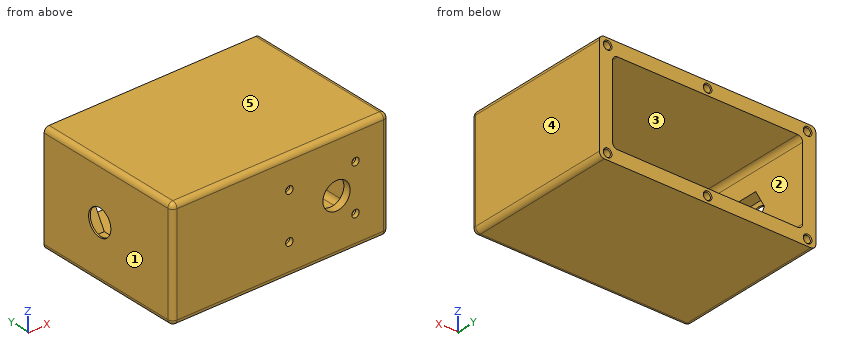
from build123d import *

# Parameters (mm, degrees)
SKETCH1_W           = 131
SKETCH1_H           = 66
BOSS_EXTRUDE1_DEPTH = 92
SKETCH10_W          = 115
SKETCH10_H          = 50
CUT_EXTRUDE7_DEPTH  = 87.5
SKETCH2_R           = 2.25
CUT_EXTRUDE1_DEPTH  = 171.801785705
SKETCH3_R           = 5
CUT_EXTRUDE2_DEPTH  = 171.801785705
SKETCH6_R           = 2.1
CUT_EXTRUDE5_DEPTH  = 7.4
CUT_EXTRUDE9_REACH  = 183.246
SKETCH17_R          = 8
SKETCH19_R          = 1.5
CUT_EXTRUDE12_DEPTH = 20
CUT_EXTRUDE13_DEPTH = 7
SKETCH7_R           = 8.25
SKETCH7_R_2         = 5
CUT_EXTRUDE14_DEPTH = 4.5
SKETCH24_R          = 3.25
CUT_EXTRUDE15_DEPTH = 2
FILLET1_R           = 3
CHAMFER1_SIZE       = 0.5


with BuildPart() as part:
    # Sketch1 → Boss-Extrude1 (new body)
    with BuildSketch(Plane(origin=(0, 0, 0), x_dir=(1, 0, 0), z_dir=(0, 1, 0))):
        with Locations((65.5, -33)):
            Rectangle(SKETCH1_W, SKETCH1_H)
    extrude(amount=BOSS_EXTRUDE1_DEPTH)

    # Sketch10 → Cut-Extrude7 (cut)
    with BuildSketch(Plane(origin=(0, 92, 0), x_dir=(1, 0, 0), z_dir=(0, 1, 0))):
        with Locations((65.5, -33)):
            Rectangle(SKETCH10_W, SKETCH10_H)
    extrude(amount=-CUT_EXTRUDE7_DEPTH, mode=Mode.SUBTRACT)

    # Sketch2 → Cut-Extrude1 (cut, through all)
    with BuildSketch(Plane(origin=(0, 4.5, 0), x_dir=(1, 0, 0), z_dir=(0, 1, 0))):
        with Locations(Location((71, -19, 0), (0, 0, 270))):
            Circle(SKETCH2_R)
        with Locations(Location((111, -19, 0), (0, 0, 270))):
            Circle(SKETCH2_R)
        with Locations(Location((71, -47, 0), (0, 0, 270))):
            Circle(SKETCH2_R)
        with Locations(Location((111, -47, 0), (0, 0, 270))):
            Circle(SKETCH2_R)
    extrude(amount=-CUT_EXTRUDE1_DEPTH, mode=Mode.SUBTRACT)

    # Sketch3 → Cut-Extrude2 (cut, through all)
    with BuildSketch(Plane(origin=(0, 4.5, 0), x_dir=(1, 0, 0), z_dir=(0, 1, 0))):
        with Locations(Location((99.54, -33, 0), (0, 0, 270))):
            Circle(SKETCH3_R)
    extrude(amount=-CUT_EXTRUDE2_DEPTH, mode=Mode.SUBTRACT)

    # Sketch6 → Cut-Extrude5 (cut)
    with BuildSketch(Plane(origin=(0, 92, 0), x_dir=(1, 0, 0), z_dir=(0, 1, 0))):
        with Locations(Location((126, -62, 0), (0, 0, 270))):
            Circle(SKETCH6_R)
        with Locations(Location((5, -62, 0), (0, 0, 270))):
            Circle(SKETCH6_R)
        with Locations(Location((5, -4, 0), (0, 0, 270))):
            Circle(SKETCH6_R)
        with Locations(Location((126, -4, 0), (0, 0, 270))):
            Circle(SKETCH6_R)
        with Locations(Location((65.5, -4, 0), (0, 0, 270))):
            Circle(SKETCH6_R)
        with Locations(Location((65.5, -62, 0), (0, 0, 270))):
            Circle(SKETCH6_R)
    extrude(amount=-CUT_EXTRUDE5_DEPTH, mode=Mode.SUBTRACT)

    # Sketch17 → Cut-Extrude9 (cut, up to next)
    with BuildSketch(Plane(origin=(0, 0, 85), x_dir=(0, 0, -1), z_dir=(1, 0, 0)), mode=Mode.PRIVATE) as cut_extrude9_sk1:
        with Locations(Location((52, 52, 0), (0, 0, 180))):
            Circle(SKETCH17_R)
    cut_extrude9_tool1 = extrude(cut_extrude9_sk1.sketch, amount=CUT_EXTRUDE9_REACH, mode=Mode.PRIVATE) & part.part
    add(cut_extrude9_tool1.solids().sort_by_distance((0, 52, 33))[0], mode=Mode.SUBTRACT)

    # Sketch19 → Cut-Extrude12 (cut)
    with BuildSketch(Plane(origin=(0, 84.6, 0), x_dir=(1, 0, 0), z_dir=(0, 1, 0))):
        with Locations(Location((5, -4, 0), (0, 0, 270))):
            Circle(SKETCH19_R)
        with Locations(Location((126, -4, 0), (0, 0, 270))):
            Circle(SKETCH19_R)
        with Locations(Location((126, -62, 0), (0, 0, 270))):
            Circle(SKETCH19_R)
        with Locations(Location((5, -62, 0), (0, 0, 270))):
            Circle(SKETCH19_R)
        with Locations(Location((65.5, -4, 0), (0, 0, 270))):
            Circle(SKETCH19_R)
        with Locations(Location((65.5, -62, 0), (0, 0, 270))):
            Circle(SKETCH19_R)
    extrude(amount=-CUT_EXTRUDE12_DEPTH, mode=Mode.SUBTRACT)

    # Sketch23 → Cut-Extrude13 (cut)
    with BuildSketch(Plane(origin=(8, 0, 0), x_dir=(0, 0, -1), z_dir=(1, 0, 0))):
        Polygon((-22.2, 58.235382907), (-33, 64.470765814), (-43.8, 58.235382907), (-43.8, 45.764617093), (-33, 39.529234186), (-22.2, 45.764617093), align=None)
    extrude(amount=-CUT_EXTRUDE13_DEPTH, mode=Mode.SUBTRACT)

    # Sketch7 → Cut-Extrude14 (cut)
    with BuildSketch(Plane(origin=(0, 4.5, 0), x_dir=(1, 0, 0), z_dir=(0, 1, 0))):
        with Locations(Location((99.54, -33, 0), (0, 0, 270))):
            Circle(SKETCH7_R)
        with Locations((99.54, -33)):
            Circle(SKETCH7_R_2, mode=Mode.SUBTRACT)
    extrude(amount=-CUT_EXTRUDE14_DEPTH, mode=Mode.SUBTRACT)

    # Sketch24 → Cut-Extrude15 (cut)
    with BuildSketch(Plane(origin=(0, 4.5, 0), x_dir=(1, 0, 0), z_dir=(0, 1, 0))):
        with Locations(Location((71, -19, 0), (0, 0, 270))):
            Circle(SKETCH24_R)
        with Locations(Location((111, -19, 0), (0, 0, 270))):
            Circle(SKETCH24_R)
        with Locations(Location((71, -47, 0), (0, 0, 270))):
            Circle(SKETCH24_R)
        with Locations(Location((111, -47, 0), (0, 0, 270))):
            Circle(SKETCH24_R)
    extrude(amount=-CUT_EXTRUDE15_DEPTH, mode=Mode.SUBTRACT)

    # Fillet1
    fillet1_edges = [part.edges().sort_by_distance(p)[0] for p in [
        (65.5, 4.5, 8),
        (8, 48.25, 8),
        (123, 4.5, 33),
        (123, 48.25, 8),
        (65.5, 4.5, 58),
        (123, 48.25, 58),
        (8, 4.5, 33),
        (8, 48.25, 58),
        (65.5, 0, 0),
        (131, 0, 33),
        (65.5, 0, 66),
        (0, 0, 33),
        (0, 46, 0),
        (131, 46, 0),
        (131, 46, 66),
        (0, 46, 66),
    ]]
    fillet(fillet1_edges, radius=FILLET1_R)

    # Chamfer1
    chamfer1_edges = [part.edges().sort_by_distance(p)[0] for p in [
        (126, 92, 1.9),
        (5, 92, 59.9),
        (65.5, 92, 1.9),
        (65.5, 92, 59.9),
        (5, 92, 1.9),
        (126, 92, 59.9),
    ]]
    chamfer(chamfer1_edges, length=CHAMFER1_SIZE)


solid = part.part
Model file for the job. Use its own axes, mm. Face numbers are marked on the shaded views. A direction names the side the tool comes from. Round coordinates to 2 decimals unless told otherwise and drop trailing zeros. Loops run counter-clockwise (first coordinate to the right, second up) from the corner with the lowest first, then second, coordinate; pieces in that order, holes last.
1. Band-saw the part on B-B, the plane x = 71. List the corners of the cut face in (y, z).
Check values:
outline: (0, 3) arc R3 ccw to (3, 0) - (92, 0) - (92, 8) - (7.5, 8) arc R3 cw to (4.5, 11) - (4.5, 15.75) - (2.5, 15.75) - (2.5, 16.75) - (0, 16.75) - close; (0, 21.25) - (2.5, 21.25) - (2.5, 22.25) - (4.5, 22.25) - (4.5, 43.75) - (2.5, 43.75) - (2.5, 44.75) - (0, 44.75) - close; (0, 49.25) - (2.5, 49.25) - (2.5, 50.25) - (4.5, 50.25) - (4.5, 55) arc R3 cw to (7.5, 58) - (92, 58) - (92, 66) - (3, 66) arc R3 ccw to (0, 63) - close
2. Mould opens along X. For the marked faces 3, 4 and 5 say: +X half, -X half, draft (parallel to the pull), parting line (faces both ways), or undercut.
Check values:
face 3: undercut
face 4: +X half
face 5: draft
3. Band-saw the part on C-C, the plane z = 19. List the corners of the cut face in (x, y).
Check values:
outline: (0, 3) arc R3 ccw to (3, 0) - (68.75, 0) - (68.75, 2.5) - (67.75, 2.5) - (67.75, 4.5) - (11, 4.5) arc R3 cw to (8, 7.5) - (8, 92) - (0, 92) - close; (73.25, 0) - (108.75, 0) - (108.75, 2.5) - (107.75, 2.5) - (107.75, 4.5) - (74.25, 4.5) - (74.25, 2.5) - (73.25, 2.5) - close; (113.25, 0) - (128, 0) arc R3 ccw to (131, 3) - (131, 92) - (123, 92) - (123, 7.5) arc R3 cw to (120, 4.5) - (114.25, 4.5) - (114.25, 2.5) - (113.25, 2.5) - close
4. Tool access for the marked faces 1 and 2: list every direction of +Z, -Z, +X, -X, +Y, -Y with a clear straight run to the whole face (end or side of a thin tool).
Check values:
face 1: +Z, -Z, -X, +Y, -Y
face 2: +Y
5. Wall check: probe 1 along Z at (x, y) = (126, 70); probe 2 along X at (y, z) = (3.6, 19); probe 3 along Z at (x, y) = (106.5, 26.5). Give the ranges that are in metal, low to high.
Check values:
probe 1: z = 0 to 2.5, 5.5 to 60.5, 63.5 to 66
probe 2: x = 0 to 67.75, 74.25 to 107.75, 114.25 to 131
probe 3: z = 0 to 8, 58 to 66
6. Band-saw the part on A-A, the plane y = 31.5. List the corners of the cut face in (x, z).
Check values:
outline: (0, 3) arc R3 ccw to (3, 0) - (128, 0) arc R3 ccw to (131, 3) - (131, 63) arc R3 ccw to (128, 66) - (3, 66) arc R3 ccw to (0, 63) - close; hole (8, 11) arc R3 ccw to (11, 8) - (120, 8) arc R3 ccw to (123, 11) - (123, 55) arc R3 ccw to (120, 58) - (11, 58) arc R3 ccw to (8, 55) - close
7. Drop flat-ended pins along their axis: P1, Ø5, axis at x = 65.5, z = 62, coming from the +Y side; P2, Ø3.5, axis at x = 65, z = 3, coming from the +Y side; P3, Ø7.5, axis at x = 111, z = 19, coming from the +Y side; P4, Ø5, axis at x = 112, z = 54, coming from the +Y side. Give the stop position or say it passes through.
Check values:
P1: stops at y = 91.9
P2: stops at y = 92
P3: stops at y = 4.5
P4: stops at y = 4.9
